```python
from build123d import *

# Parameters (mm, degrees)
SKETCH_1_W          = 29
SKETCH_1_H          = 4
SKETCH_1_W_2        = 4
SKETCH_1_H_2        = 16
EXTRUDE_1_DEPTH     = 55
SKETCH_3_R          = 2.75
CUT_EXTRUDE_3_DEPTH = 20
SKETCH_2_R          = 2.75
CUT_EXTRUDE_4_DEPTH = 20
FILLET_2_R          = 1
CUT_EXTRUDE_START   = -3
CUT_EXTRUDE_5_DEPTH = 3
CUT_EXTRUDE_6_DEPTH = 3
FILLET_3_R          = 3


with BuildPart() as part:
    # 스케치1 → 보스-돌출1 (new, symmetric)
    with BuildSketch(Plane.XY):
        with Locations((14.5, -2)):
            Rectangle(SKETCH_1_W, SKETCH_1_H)
        with Locations((2, 8)):
            Rectangle(SKETCH_1_W_2, SKETCH_1_H_2)
    extrude(amount=EXTRUDE_1_DEPTH, both=True)

    # 스케치3 → 컷-돌출3 (cut)
    with BuildSketch(Plane(origin=(4, 0, 0), x_dir=(0, 0, -1), z_dir=(1, 0, 0))):
        with Locations(Location((0, 6, 0), (0, 0, 90))):
            Circle(SKETCH_3_R)
        with Locations(Location((-45, 6, 0), (0, 0, 90))):
            Circle(SKETCH_3_R)
        with Locations(Location((45, 6, 0), (0, 0, 90))):
            Circle(SKETCH_3_R)
    extrude(amount=-CUT_EXTRUDE_3_DEPTH, mode=Mode.SUBTRACT)

    # 스케치2 → 컷-돌출4 (cut)
    with BuildSketch(Plane(origin=(0, 0, 0), x_dir=(1, 0, 0), z_dir=(0, 1, 0))):
        with Locations(Location((19, 0, 0), (0, 0, 180))):
            Circle(SKETCH_2_R)
        with Locations(Location((19, -45, 0), (0, 0, 180))):
            Circle(SKETCH_2_R)
        with Locations(Location((19, 45, 0), (0, 0, 180))):
            Circle(SKETCH_2_R)
    extrude(amount=-CUT_EXTRUDE_4_DEPTH, mode=Mode.SUBTRACT)

    # 필렛2
    fillet_2_edges = [part.edges().sort_by_distance(p)[0] for p in [
        (0, -4, 0),
        (4, 0, 0),
    ]]
    fillet(fillet_2_edges, radius=FILLET_2_R)

    # 스케치4 → 컷-돌출5 (cut)
    with BuildSketch(Plane.XY.offset(55).offset(CUT_EXTRUDE_START)):
        with BuildLine():
            Line((0, 16), (0, -3))
            ThreePointArc((0, -3), (0.292893219, -3.707106781), (1, -4))
            Line((1, -4), (29, -4))
            Line((29, -4), (29, 0))
            Line((29, 0), (5, 0))
            ThreePointArc((5, 0), (4.292893219, 0.292893219), (4, 1))
            Line((4, 1), (4, 16))
            Line((4, 16), (0, 16))
        make_face()
    extrude(amount=CUT_EXTRUDE_5_DEPTH, mode=Mode.SUBTRACT)

    # 스케치5 → 컷-돌출6 (cut)
    with BuildSketch(Plane(origin=(0, 0, -55), x_dir=(-1, 0, 0), z_dir=(0, 0, -1))):
        with BuildLine():
            Line((-29, -4), (-1, -4))
            ThreePointArc((-1, -4), (-0.292893219, -3.707106781), (0, -3))
            Line((0, -3), (0, 16))
            Line((0, 16), (-4, 16))
            Line((-4, 16), (-4, 1))
            ThreePointArc((-4, 1), (-4.292893219, 0.292893219), (-5, 0))
            Line((-5, 0), (-29, 0))
            Line((-29, 0), (-29, -4))
        make_face()
    extrude(amount=-CUT_EXTRUDE_6_DEPTH, mode=Mode.SUBTRACT)

    # 필렛3
    fillet_3_edges = [part.edges().sort_by_distance(p)[0] for p in [
        (29, -2, -52),
        (2, 16, -52),
        (2, 16, 52),
        (29, -2, 52),
    ]]
    fillet(fillet_3_edges, radius=FILLET_3_R)


solid = part.part
```
CAD build for the part. Positions are in the model's coordinates, mm. A direction names the side the tool comes from. Round coordinates to 2 decimals unless told otherwise and drop trailing zeros. Write each loop counter-clockwise with the first axis right and the second up, starting at its lowest first coordinate (ties: lowest second). Pieces come first, ordered by that corner, then holes. Notation, with made-up numbers: (1.25, 84) - (8.25, 84) arc R27 cw to (8.25, 119) - close; hole circle Ø4 at (31, 45.25). An arc over 180 degrees is marked (long way). Return JSON: item names as keys, results as strings. Group by question number.
Item 1: 3-axis set-ups, long thin cutter, end or side, ignore diameter. For faces 1 (the face through (21.747, -1.972, 0.121)), 2 (the face through (4, 10, 1)): which of +Z, -Z, +X, -X, +Y, -Y reach the whole face in a straight line?
Item 2: Band-saw the part on B-B on z = -45. List the corners of the cut face in (x, y), plus the area to 3 significant figures.
Item 3: Probe probe 1 along Z at (x, y) = (19, -1.25); probe 2 along Z at (x, y) = (1.5, 3.5); probe 3 along Y at (x, z) = (16.75, 18). List the from-to ranges inside material, lowest first.
Item 4: Band-saw the part on A-A on x = 19. List the corners of the cut face in (y, z), plus the area to 3 significant figures.
Item 5: Flat gauge pins, fed straight in: pin 1 Ø2 at (x, z) = (9, -7) entering from +Y; pin 2 Ø3.5 at (x, z) = (19, 0) entering from +Y; pin 3 Ø7 at (y, z) = (6, -45) entering from +X. Where does each tip first touch, or does it go through?
Item 6: Band-saw the part on C-C on y = 6. List the corners of the cut face in (x, z), plus the area to 3 significant figures.
Item 7: Mould opens along Y. For faces 3 (the face through (28.14, -2.03, -51.1)), 4 (the face through (2.028, 5.642, 47.727)), 5 (the face through (2.028, 5.642, -42.273)), 6 (the face through (14, 0, 1)) say: +Y half, -Y half, draft (parallel to the pull), parting line (faces both ways), or undercut.
Item 8: Band-saw the part on D-D on x = 2. List the corners of the cut face in (y, z).
Resolved:
{
 "1": {"face 1": "+Y, -Y", "face 2": "+Z, -Z, +X, +Y"},
 "2": {"outline": "(0, -3) arc R1 ccw to (1, -4) - (16.25, -4) - (16.25, 0) - (5, 0) arc R1 cw to (4, 1) - (4, 3.25) - (0, 3.25) - close; (0, 8.75) - (4, 8.75) - (4, 16) - (0, 16) - close; (21.75, -4) - (29, -4) - (29, 0) - (21.75, 0) - close", "area": "136 mm²"},
 "3": {"probe 1": "z = -52 to -47.75, -42.25 to -2.75, 2.75 to 42.25, 47.75 to 52", "probe 2": "z = -52 to -46.15, -43.85 to -1.15, 1.15 to 43.85, 46.15 to 52", "probe 3": "y = -4 to 0"},
 "4": {"outline": "(-4, -52) - (0, -52) - (0, -47.75) - (-4, -47.75) - close; (-4, -42.25) - (0, -42.25) - (0, -2.75) - (-4, -2.75) - close; (-4, 2.75) - (0, 2.75) - (0, 42.25) - (-4, 42.25) - close; (-4, 47.75) - (0, 47.75) - (0, 52) - (-4, 52) - close", "area": "350 mm²"},
 "5": {"pin 1": "stops at y = 0", "pin 2": "passes through", "pin 3": "stops at x = 4"},
 "6": {"outline": "(0, -52) - (4, -52) - (4, -47.75) - (0, -47.75) - close; (0, -42.25) - (4, -42.25) - (4, -2.75) - (0, -2.75) - close; (0, 2.75) - (4, 2.75) - (4, 42.25) - (0, 42.25) - close; (0, 47.75) - (4, 47.75) - (4, 52) - (0, 52) - close", "area": "350 mm²"},
 "7": {"face 3": "draft", "face 4": "undercut", "face 5": "undercut", "face 6": "+Y half"},
 "8": {"outline": "(-4, -52) - (13, -52) arc R3 ccw to (16, -49) - (16, 49) arc R3 ccw to (13, 52) - (-4, 52) - close; hole circle Ø5.5 at (6, -45); hole circle Ø5.5 at (6, 0); hole circle Ø5.5 at (6, 45)"}
}
